Work out the finished part from the listing and answer in its coordinate system (mm). A direction names the side the tool comes from. Give positions to 0.01 mm unless a question says otherwise; leave off trailing zeros. Loops run counter-clockwise (first coordinate to the right, second up) from the corner with the lowest first, then second, coordinate; pieces in that order, holes last. Notation, with made-up numbers: (14, -26) - (43, -26) arc R20 ccw to (43, -4) - close; hole circle Ø4 at (-37.75, -37). An arc over 180 degrees is marked (long way). One line per question, with ' | ' between items.
from build123d import *

# Parameters (mm, degrees)
SKETCH1_R           = 2.5
BOSS_EXTRUDE1_DEPTH = 15
SKETCH2_R           = 4.159584877
BOSS_EXTRUDE2_DEPTH = 2.8
FILLET1_R           = 2.5
CUT_EXTRUDE1_DEPTH  = 2


with BuildPart() as part:
    # Sketch1 → Boss-Extrude1 (new body)
    with BuildSketch(Plane.XY):
        Circle(SKETCH1_R)
    extrude(amount=BOSS_EXTRUDE1_DEPTH)

    # Sketch2 → Boss-Extrude2 (add)
    with BuildSketch(Plane(origin=(0, 0, 0), x_dir=(-1, 0, 0), z_dir=(0, 0, -1))):
        Circle(SKETCH2_R)
    extrude(amount=BOSS_EXTRUDE2_DEPTH)

    # Fillet1
    fillet1_edges = [part.edges().sort_by_distance(p)[0] for p in [
        (4.159584877, 0, -2.8),
    ]]
    fillet(fillet1_edges, radius=FILLET1_R)

    # Sketch3 → Cut-Extrude1 (cut)
    with BuildSketch(Plane(origin=(0, 0, -2.8), x_dir=(-1, 0, 0), z_dir=(0, 0, -1))):
        Polygon((1.392434699, -0.636521364), (1.247461021, 0.88762314), (-0.144973678, 1.524144504), (-1.392434699, 0.636521364), (-1.247461021, -0.88762314), (0.144973678, -1.524144504), align=None)
    extrude(amount=-CUT_EXTRUDE1_DEPTH, mode=Mode.SUBTRACT)


solid = part.part
1. Consider L1, parallel to Z at x = 0.5, y = 0.25; L2, parallel to Y at x = 0, z = 3.5; L3, parallel to Z at x = -2, y = -0.75. Determine where each line is inside the solid, lowest interval first.
Evaluation:
L1: -0.8 to 15 | L2: -2.5 to 2.5 | L3: -2.75 to 15
2. Which of the six approach directions +Z, -Z, +X, -X, +Y, -Y give full straight-line access (tool end or side, diameter ignored) to faces 4 (the flat face through (1, -1, -2)), 5 (the flat face through (-2, -2, 0)), 6 (the cylindrical face through (-1.92, -3.69, -0.15))?
Evaluation:
face 4: -Z | face 5: +Z | face 6: +Z, -Z
3. A flat-ended cylindrical pin translates along its axis: pin 1 (4 mm diameter, centred on x = 3, z = 6, fed in from -Y). Find the tip coordinate at first contact, or state that the pin passes through.
Evaluation:
pin 1: y = -2.29
4. Determine the mould class of faces 1 (the flat face through (0, 0, 15)), 2 (the cylindrical face through (-0.54, -2.44, 7.4)), 3 (the flat face through (0.76, 1.087, -1.814)) for opening direction X: +X half, -X half, draft (parallel to the pull), parting line (faces both ways), or undercut.
Evaluation:
face 1: draft | face 2: parting line | face 3: undercut
5. Find section A-A on z = 12. Write down the section's boundary in (x, y).
Evaluation:
outline: circle Ø5 at (0, 0)
